```python
from build123d import *

# Parameters (mm, degrees)
SKETCH_1_R          = 3
EXTRUDE_1_DEPTH     = 10
SKETCH_2_W          = 1
SKETCH_2_H          = 0.5
SKETCH_3_R          = 1.5
CUT_EXTRUDE_1_DEPTH = 2
SKETCH_4_W          = 4.889658543
SKETCH_4_H          = 6.2
EXTRUDE_2_DEPTH     = 0.5


with BuildPart() as part:
    # Эскиз1 → Бобышка-Вытянуть1 (new body)
    with BuildSketch(Plane(origin=(0, 0, 0), x_dir=(0, 0, -1), z_dir=(1, 0, 0))):
        Circle(SKETCH_1_R)
    extrude(amount=EXTRUDE_1_DEPTH)

    # Эскиз2 → Вырез-Повернуть1 (revolve, cut)
    with BuildSketch(Plane.XY, mode=Mode.PRIVATE) as cut_revolve_1_sk:
        with Locations((3.5, 2.75)):
            Rectangle(SKETCH_2_W, SKETCH_2_H)
    revolve(cut_revolve_1_sk.sketch.rotate(Axis((-1000, 0, 0), (1, 0, 0)), 90), axis=Axis((-1000, 0, 0), (1, 0, 0)), mode=Mode.SUBTRACT)

    # Эскиз3 → Вырез-Вытянуть1 (cut)
    with BuildSketch(Plane(origin=(10, 0, 0), x_dir=(0, 0, -1), z_dir=(1, 0, 0))):
        Circle(SKETCH_3_R)
    extrude(amount=-CUT_EXTRUDE_1_DEPTH, mode=Mode.SUBTRACT)

    # Эскиз4 → Бобышка-Вытянуть2 (add, symmetric)
    with BuildSketch(Plane.XY):
        with Locations((-0.555170728, 0)):
            Rectangle(SKETCH_4_W, SKETCH_4_H)
    extrude(amount=EXTRUDE_2_DEPTH, both=True)


solid = part.part
```
Here's how the part is built. I have some questions about the finished solid (model axes, mm). A direction names the side the tool comes from. Coordinates: 2 decimals unless noted, no trailing zeros. Loops run counter-clockwise (first coordinate to the right, second up) from the corner with the lowest first, then second, coordinate; pieces in that order, holes last. Notation, with made-up numbers: (-35.75, 40.25) -> (-23.75, 40.25) arc R25 ccw to (-23.75, 72.25) -> close; hole circle Ø10 at (0, 62). An arc over 180 degrees is marked (long way). Return JSON: item names as keys, results as strings.
1) For faces 4 (the face through (9.01, 0.07, 1.5)), 5 (the face through (3, -2, 2)), 6 (the face through (10, -1.3, -1.3)), 7 (the face through (-1, -3.1, 0)), 8 (the face through (0, 0, 1)), which set-ups out of +Z, -Z, +X, -X, +Y, -Y let a thin tool reach every point of the face, with its end or its side?
Results below:
{"face 4": "+X", "face 5": "none", "face 6": "+Z, -Z, +X, +Y, -Y", "face 7": "+Z, -Z, +X, -X, -Y", "face 8": "+Z, -X, +Y, -Y"}
2) If we section it at C-C, the plane z = 0: Write out the boundary of the cut face in (x, y), then the cut area to 3 significant figures.
Results below:
{"outline": "(-3, -3.1) -> (1.89, -3.1) -> (1.89, -3) -> (3, -3) -> (3, -2.5) -> (4, -2.5) -> (4, -3) -> (10, -3) -> (10, -1.5) -> (8, -1.5) -> (8, 1.5) -> (10, 1.5) -> (10, 3) -> (4, 3) -> (4, 2.5) -> (3, 2.5) -> (3, 3) -> (1.89, 3) -> (1.89, 3.1) -> (-3, 3.1) -> close", "area": "72.0 mm²"}
3) I need wall thicknesses on line 1 (X direction, y = 2.75, z = -1.1); line 2 (Y direction, x = 9.35, z = 0); line 3 (X direction, y = 2, z = -0.85). Which ranges of each line are inside material? Lowest first, please. Write a range as from..to.
Results below:
{"line 1": "0..3, 4..10", "line 2": "-3..-1.5, 1.5..3", "line 3": "0..10"}
4) If we section it at D-D, the plane x = 8.5: Write out the boundary of the cut face in (y, z).
Results below:
{"outline": "circle Ø6 at (0, 0); hole circle Ø3 at (0, 0)"}
5) If we section it at A-A, the plane x = 1.5: Write out the boundary of the cut face in (y, z), then the cut area to 3 significant figures.
Results below:
{"outline": "(-3.1, -0.5) -> (-2.96, -0.5) arc R3 ccw to (2.96, -0.5) -> (3.1, -0.5) -> (3.1, 0.5) -> (2.96, 0.5) arc R3 ccw to (-2.96, 0.5) -> (-3.1, 0.5) -> close", "area": "28.5 mm²"}
6) If we section it at B-B, the plane y = 0: Write out the boundary of the cut face in (x, z).
Results below:
{"outline": "(-3, -0.5) -> (0, -0.5) -> (0, -3) -> (3, -3) -> (3, -2.5) -> (4, -2.5) -> (4, -3) -> (10, -3) -> (10, -1.5) -> (8, -1.5) -> (8, 1.5) -> (10, 1.5) -> (10, 3) -> (4, 3) -> (4, 2.5) -> (3, 2.5) -> (3, 3) -> (0, 3) -> (0, 0.5) -> (-3, 0.5) -> close"}
7) Will these pins go through, and if not, where does the flat tip stop? pin 1 (2.5 mm diameter, centred on y = 0, z = 0, fed in from +X); pin 2 (1 mm diameter, centred on x = 6.5, z = -0.5, fed in from +Y); pin 3 (1.3 mm diameter, centred on y = 0, z = -1.5, fed in from -X).
Results below:
{"pin 1": "x = 8", "pin 2": "y = 3", "pin 3": "x = 0"}
8) Thinking about a two-plate mould opening in X: for faces 1 (the face through (-1, 3.1, 0)), 2 (the face through (0, 0, -1)), 3 (the face through (4, -2, 2)), which applies, +X half, -X half, draft (parallel to the pull), parting line (faces both ways), or undercut?
Results below:
{"face 1": "draft", "face 2": "-X half", "face 3": "undercut"}
